Read the model definition and answer for the solid it produces. Units are mm, in the model's axes. Coordinates: 2 decimals unless noted, no trailing zeros. Write each loop counter-clockwise with the first axis right and the second up, starting at its lowest first coordinate (ties: lowest second). Pieces come first, ordered by that corner, then holes.
1) The part is cut by section A-A (z = -26.5). Determine the outline of the cut face in (x, y).
2) Find the intervals of material crossed by line 1 (Z direction, x = 0, y = -0.75) (3 decimals); line 2 (Z direction, x = 0, y = 4.35) (3 decimals); line 3 (Y direction, x = -29, z = -9), in increasing order.
3) The part is cut by section C-C (x = -11.5). Determine the outline of the cut face in (y, z).
4) The part is cut by section D-D (x = -34.5). Determine the outline of the cut face in (y, z).
5) The part is cut by section B-B (y = -3.5). Determine the outline of the cut face in (x, z) (3 decimals), then the cut area to 3 significant figures.
6) Each of these flat-tipped pins is pushed along its axis until it touches: pin 1 Ø10.5 at (x, z) = (0, 0) entering from +Y; pin 2 Ø1.5 at (y, z) = (1.5, 33) entering from +X; pin 3 Ø10 at (x, z) = (-15, -40.5) entering from -Y. Where does it stop, or does it pass through?
Autodesk Inventor part; units mm, degrees
ref_plane "YZ Plane" through (0, 0, 0) normal (1, 0, 0) x (0, 1, 0)
ref_plane "XZ Plane" through (0, 0, 0) normal (0, 1, 0) x (-1, 0, 0)
ref_plane "XY Plane" through (0, 0, 0) normal (0, 0, 1) x (1, 0, 0)
sketch "Sketch1" plane through (0, 0, 0) normal (0, 1, 0) x (-1, 0, 0)
  circle A0 centre (0, 0) radius 53
  dimension "d0" = 106
extrude "Extrusion1" add sketch "Sketch1" along normal blind 5
sketch "Sketch2" plane through (0, 5, 0) normal (0, 1, 0) x (1, 0, 0)
  line L0 (13, -30.5) -> (13, 30.5) construction
  line L1 (13, 30.5) -> (-13, 30.5) construction
  line L2 (-13, 30.5) -> (-13, -30.5) construction
  line L3 (-13, -30.5) -> (13, -30.5) construction
  line L4 (13, -30.5) -> (-13, 30.5) construction
  line L5 (13, 30.5) -> (-13, -30.5) construction
  line L6 (-13, -30.5) -> (-10.25, -30.5)
  line L7 (-13, 30.5) -> (-10.25, 30.5)
  line L8 (13, -30.5) -> (10.25, -30.5) construction
  line L9 (13, 30.5) -> (10.25, 30.5)
  line L10 (10.25, -36.5) -> (10.25, -24.5) construction
  line L11 (13, -36.5) -> (13, -24.5)
  line L12 (7.5, -24.5) -> (7.5, -36.5)
  arc A0 (7.5, -36.5) -> (13, -36.5) centre (10.25, -36.5) ccw
  arc A1 (13, -24.5) -> (7.5, -24.5) centre (10.25, -24.5) ccw
  line L13 (-7.5, -36.5) -> (-7.5, -24.5)
  line L14 (-13, -24.5) -> (-13, -36.5)
  arc A2 (-13, -36.5) -> (-7.5, -36.5) centre (-10.25, -36.5) ccw
  arc A3 (-7.5, -24.5) -> (-13, -24.5) centre (-10.25, -24.5) ccw
  line L15 (13, 24.5) -> (13, 36.5)
  line L16 (7.5, 36.5) -> (7.5, 24.5)
  arc A4 (7.5, 24.5) -> (13, 24.5) centre (10.25, 24.5) ccw
  arc A5 (13, 36.5) -> (7.5, 36.5) centre (10.25, 36.5) ccw
  line L17 (-7.5, 24.5) -> (-7.5, 36.5)
  line L18 (-13, 36.5) -> (-13, 24.5)
  arc A6 (-13, 24.5) -> (-7.5, 24.5) centre (-10.25, 24.5) ccw
  arc A7 (-7.5, 36.5) -> (-13, 36.5) centre (-10.25, 36.5) ccw
  point P0 (0, 0)
  point P1 (0, 0)
  dimension "d3" = 61
  dimension "d4" = 26
  dimension "d5" = 2.75
  dimension "d6" = 2.75
  dimension "d7" = 2.75
  dimension "d8" = 2.75
  dimension "d9" = 6
  dimension "d10" = 5.5
  dimension "d11" = 6
  dimension "d12" = 5.5
  dimension "d13" = 6
  dimension "d14" = 5.5
  dimension "d15" = 6
  dimension "d16" = 5.5
extrude "Extrusion2" cut sketch "Sketch2" against normal through all
sketch "Sketch3" plane through (0, 0, 0) normal (0, -1, 0) x (1, 0, 0)
  circle A0 centre (0, 0) radius 7.275
  line L0 (7.275, 0) -> (-7.275, 0) construction
  line L1 (0, 7.275) -> (0, -7.275) construction
  line L2 (9.775, 2.5) -> (4.775, 2.5)
  line L3 (4.775, 2.5) -> (4.775, -2.5)
  line L4 (4.775, -2.5) -> (9.775, -2.5)
  line L5 (9.775, -2.5) -> (9.775, 2.5)
  line L6 (9.775, 2.5) -> (4.775, -2.5) construction
  line L7 (4.775, 2.5) -> (9.775, -2.5) construction
  line L8 (2.5, 9.775) -> (-2.5, 9.775)
  line L9 (-2.5, 9.775) -> (-2.5, 4.775)
  line L10 (-2.5, 4.775) -> (2.5, 4.775)
  line L11 (2.5, 4.775) -> (2.5, 9.775)
  line L12 (2.5, 9.775) -> (-2.5, 4.775) construction
  line L13 (-2.5, 9.775) -> (2.5, 4.775) construction
  line L14 (-9.775, 2.5) -> (-4.775, 2.5)
  line L15 (-4.775, 2.5) -> (-4.775, -2.5)
  line L16 (-4.775, -2.5) -> (-9.775, -2.5)
  line L17 (-9.775, -2.5) -> (-9.775, 2.5)
  line L18 (-9.775, 2.5) -> (-4.775, -2.5) construction
  line L19 (-4.775, 2.5) -> (-9.775, -2.5) construction
  line L20 (-2.5, -4.775) -> (2.5, -4.775)
  line L21 (2.5, -4.775) -> (2.5, -9.775)
  line L22 (2.5, -9.775) -> (-2.5, -9.775)
  line L23 (-2.5, -9.775) -> (-2.5, -4.775)
  line L24 (-2.5, -4.775) -> (2.5, -9.775) construction
  line L25 (2.5, -4.775) -> (-2.5, -9.775) construction
  point P0 (6.832, 2.5)
  point P1 (2.5, 6.832)
  point P2 (-2.5, 6.832)
  point P3 (-6.832, 2.5)
  point P4 (-6.832, -2.5)
  point P5 (-2.5, -6.832)
  point P6 (2.5, -6.832)
  point P7 (6.832, -2.5)
  dimension "d20" = 14.55
  dimension "d21" = 5
  dimension "d22" = 5
  dimension "d23" = 5
  dimension "d24" = 5
  dimension "d25" = 5
  dimension "d26" = 5
  dimension "d27" = 5
  dimension "d28" = 5
extrude "Extrusion3" add sketch "Sketch3" along normal blind 5 contours L2 L3 L4 A0 L21 L20 L23 L16 L15 L14 L9 L10 L11
hole "Hole1" at (0, 5, 0) direction (0, -1, 0) diameter 6.6 end through all counterbore diameter 14.55 counterbore depth 3
properties part number "BaseGear" material "ABS Plastic"
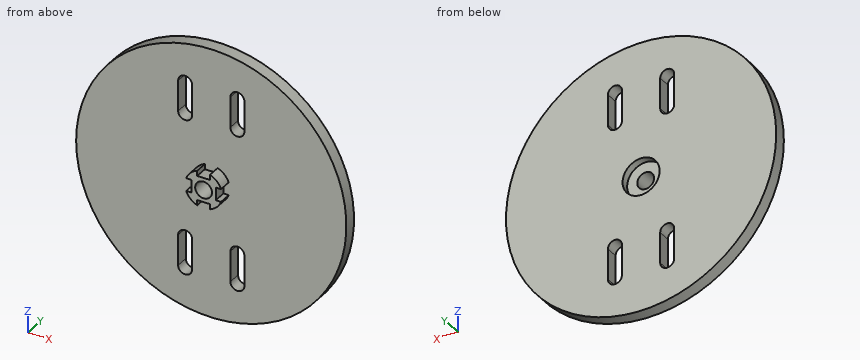
Reported:
1. outline: (-45.9, 0) - (-13, 0) - (-13, 5) - (-45.9, 5) - close; (-7.5, 0) - (7.5, 0) - (7.5, 5) - (-7.5, 5) - close; (13, 0) - (45.9, 0) - (45.9, 5) - (13, 5) - close
2. line 1: z = -4.775 to -3.3, 3.3 to 4.775
2. line 2: z = -53 to -7.275, 7.275 to 53
2. line 3: y = 0 to 5
3. outline: (0, -51.74) - (5, -51.74) - (5, -38.95) - (0, -38.95) - close; (0, -22.05) - (5, -22.05) - (5, 22.05) - (0, 22.05) - close; (0, 38.95) - (5, 38.95) - (5, 51.74) - (0, 51.74) - close
4. outline: (0, -40.23) - (5, -40.23) - (5, 40.23) - (0, 40.23) - close
5. outline: (-6.832, -2.5) arc R7.275 ccw to (-2.5, -6.832) - (-2.5, -4.775) - (2.5, -4.775) - (2.5, -6.832) arc R7.275 ccw to (6.832, -2.5) - (4.775, -2.5) - (4.775, 2.5) - (6.832, 2.5) arc R7.275 ccw to (2.5, 6.832) - (2.5, 4.775) - (-2.5, 4.775) - (-2.5, 6.832) arc R7.275 ccw to (-6.832, 2.5) - (-4.775, 2.5) - (-4.775, -2.5) - close; hole circle Ø6.6 at (0, 0)
5. area: 85.0 mm2
6. pin 1: stops at y = 2
6. pin 2: stops at x = 42.06
6. pin 3: stops at y = 0
